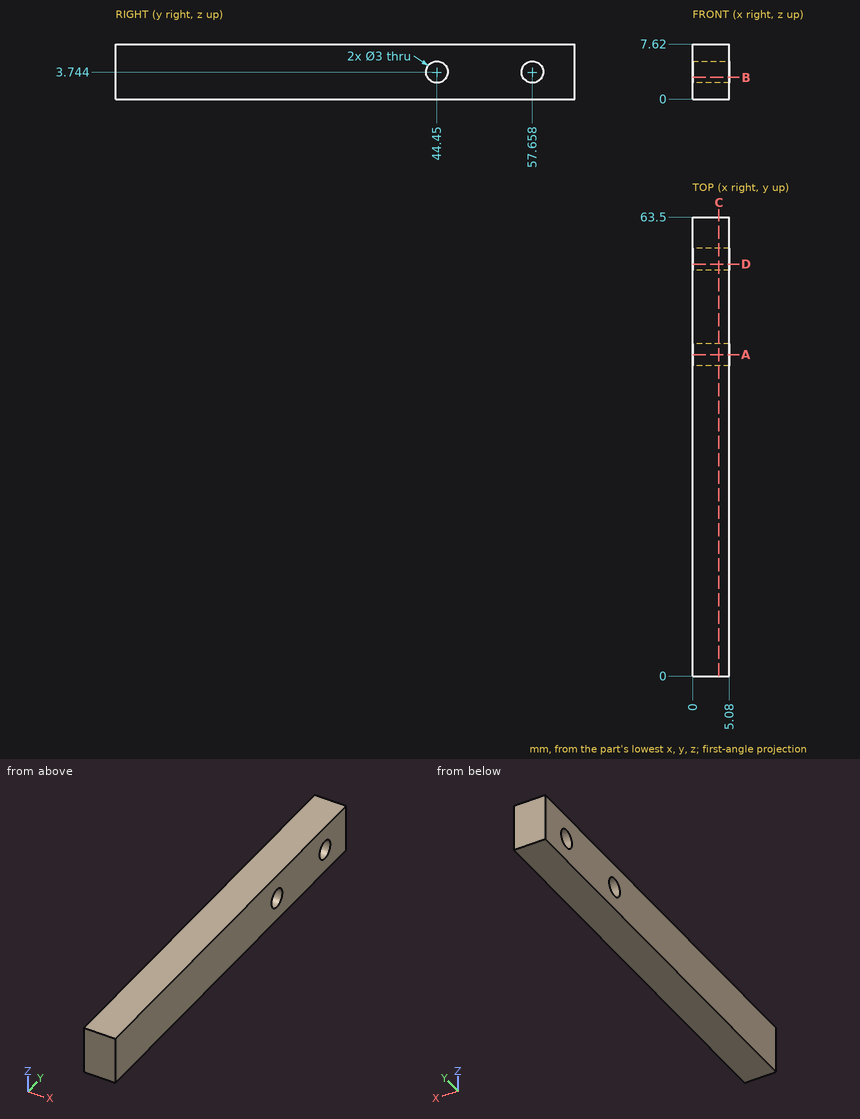
Can you work these out from the drawing? Everything is in mm from the part's minimum corner. Round coordinates to 2 decimals unless told otherwise and drop trailing zeros. Write each loop counter-clockwise with the first axis right and the second up, starting at its lowest first coordinate (ties: lowest second). Pieces come first, ordered by that corner, then holes. Notation, with made-up numbers: (54.25, 34) - (63.25, 34) arc R16 cw to (63.25, 40) - close; hole circle Ø5 at (34.5, 40). An arc over 180 degrees is marked (long way). Put each result on its own line as item: value. Start each with the question number.
(1) I want a section at A-A, the plane y = 44.45. Please give me the cut outline in (x, z) (1 decimal).
(2) I want a section at C-C, the plane x = 3.65. Give the number of separate pieces and of enclosed holes in the cut face, plus the area to 3 significant figures.
(3) I want a section at D-D, the plane y = 57. Please give me the cut outline in (x, z).
(4) Will these pins go through, and if not, where does the flat tip stop? pin 1 (3 mm diameter, centred on y = 47.5, z = 1, fed in from -X); pin 2 (2.5 mm diameter, centred on y = 57.66, z = 3.74, fed in from +X).
(5) I need wall thicknesses on probe 1 along Y at (x, z) = (4.05, 3) (1 decimal); probe 2 along Y at (x, z) = (0.2, 4.75) (1 decimal); probe 3 along Z at (x, y) = (1.65, 57.5) (1 decimal). Which ranges of each line are inside material? Lowest first, please.
(6) I want a section at B-B, the plane z = 3. Please give me the cut outline in (x, y) (1 decimal).
Here are the results:
1. outline: (0, 0) - (5.1, 0) - (5.1, 2.2) - (0, 2.2) - close; (0, 5.2) - (5.1, 5.2) - (5.1, 7.6) - (0, 7.6) - close
2. separate pieces: 1
2. enclosed holes: 2
2. area: 470 mm^2
3. outline: (0, 0) - (5.08, 0) - (5.08, 2.4) - (0, 2.4) - close; (0, 5.09) - (5.08, 5.09) - (5.08, 7.62) - (0, 7.62) - close
4. pin 1: stops at x = 0
4. pin 2: passes through
5. probe 1: y = 0 to 43.1, 45.8 to 56.4, 59 to 63.5
5. probe 2: y = 0 to 43.3, 45.6 to 56.5, 58.8 to 63.5
5. probe 3: z = 0 to 2.3, 5.2 to 7.6
6. outline: (0, 0) - (5.1, 0) - (5.1, 43.1) - (0, 43.1) - close; (0, 45.8) - (5.1, 45.8) - (5.1, 56.4) - (0, 56.4) - close; (0, 59) - (5.1, 59) - (5.1, 63.5) - (0, 63.5) - close
